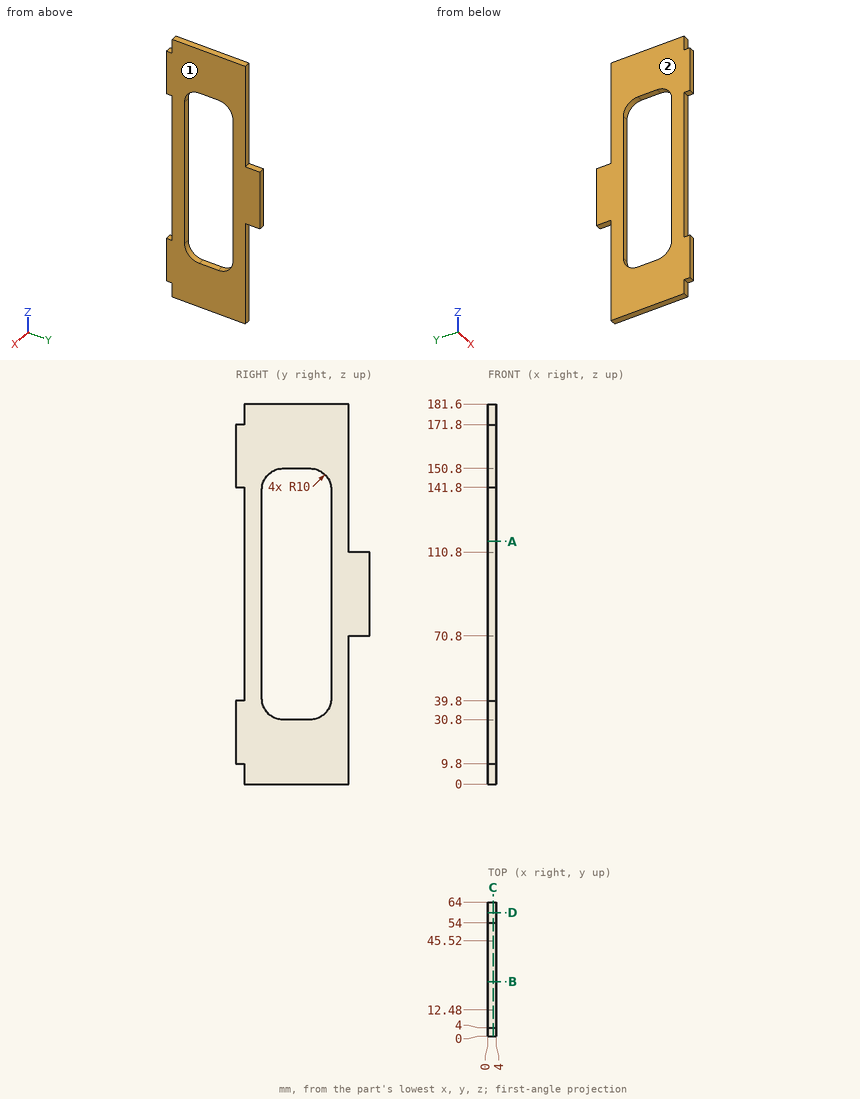
Input: dimensioned drawing with shaded views. Units: mm. Origin: part minimum x, y, z. Coordinates: 2 decimals unless noted, no trailing zeros. Loops run counter-clockwise (first coordinate to the right, second up) from the corner with the lowest first, then second, coordinate; pieces in that order, holes last. Notation, with made-up numbers: M 36,9.25 L 64,9.25 A21 ccw 64,27.25 Z; hole C 56,29.25 d1. An arc over 180 degrees is marked long. One line per item, written item: value.
(1) Pin query (flat end, axial travel): pin 1 (1.2 mm diameter, centred on x = 2.5, z = 4.5, fed in from -Y); pin 2 (1.2 mm diameter, centred on x = 1.5, y = 59.5, fed in from -Z); pin 3 (2 mm diameter, centred on x = 2, y = 2.5, fed in from -Z); pin 4 (1.2 mm diameter, centred on x = 2.5, y = 26.5, fed in from -Z). Return the tip coordinate at first contact, or that it passes through.
Filled in:
pin 1: y = 4
pin 2: z = 70.8
pin 3: z = 9.8
pin 4: z = 0
(2) Section C-C (x = 2.55). Output: boundary loops of the cut face in (y, z), and give its area (3 significant figures).
Filled in:
outline: M 0,9.8 L 4,9.8 L 4,0 L 54,0 L 54,70.8 L 64,70.8 L 64,110.8 L 54,110.8 L 54,181.6 L 4,181.6 L 4,171.8 L 0,171.8 L 0,141.8 L 4,141.8 L 4,39.8 L 0,39.8 Z; hole M 12.48,40.8 A10 ccw 22.48,30.8 L 35.52,30.8 A10 ccw 45.52,40.8 L 45.52,140.8 A10 ccw 35.52,150.8 L 22.48,150.8 A10 ccw 12.48,140.8 Z
area: 5,840 mm^2
(3) Section D-D (y = 59). Output: boundary loops of the cut face in (x, z), and give its area (3 significant figures).
Filled in:
outline: M 0,70.8 L 4,70.8 L 4,110.8 L 0,110.8 Z
area: 160 mm^2
(4) Pull-direction query (X, two-part tool) for the marked faces 1 and 2; classes: +X half, -X half, draft (parallel to the pull), parting line (faces both ways), or undercut.
Filled in:
face 1: +X half
face 2: -X half
(5) Section A-A (z = 116). Output: boundary loops of the cut face in (x, y).
Filled in:
outline: M 0,4 L 4,4 L 4,12.48 L 0,12.48 Z; M 0,45.52 L 4,45.52 L 4,54 L 0,54 Z
(6) Section B-B (y = 26). Output: boundary loops of the cut face in (x, z), and give its area (3 significant figures).
Filled in:
outline: M 0,0 L 4,0 L 4,30.8 L 0,30.8 Z; M 0,150.8 L 4,150.8 L 4,181.6 L 0,181.6 Z
area: 246 mm^2
(7) Line query: line 1 along Y through (x, z) = (2.75, 44); line 2 along Y through (x, z) = (3.65, 109); line 3 along Y through (x, z) = (3.85, 159). Output: solid intervals per line, ascending. Write a range as from..to.
Filled in:
line 1: 4..12.48, 45.52..54
line 2: 4..12.48, 45.52..64
line 3: 0..54
